from build123d import *

# Parameters (mm, degrees)
F2_R = 1.99999
F3_R = 9


# Not quite as in the source:
# - a fillet or chamfer is up to 0.001 mm smaller than in the source, because OpenCascade refuses the exact size


with BuildPart() as f1:
    # F0 (on Front) → F1 (revolve)
    with BuildSketch(Plane.XZ):
        Polygon((-9.5, -13.2402114049), (-7.5, 23.7597885951), (0, 23.7597885951), (0, 28.8208965212), (-11.5044763215, 28.8208965212), (-11.5044763215, 23.7850059011), (-13.4568578627, -12.3340526108), align=None)
    revolve(axis=Axis((0, 0, 3.3093634993), (0, 0, -1)))

    # F2 (radius 2 in the source; OpenCascade refuses exactly that, so slightly less here)
    f2_edges = [f1.edges().sort_by_distance(p)[0] for p in [
        (9.5, 0, -13.240211),
        (13.456858, 0, -12.334053),
    ]]
    fillet(f2_edges, radius=F2_R)

    # F3
    f3_edges = [f1.edges().sort_by_distance(p)[0] for p in [
        (11.504476, 0, 28.820897),
    ]]
    fillet(f3_edges, radius=F3_R)


solid = f1.part
Check sheet for the modelled part. Datum: model origin and axes. Units: mm. Give positions to 0.01 mm unless a question says otherwise; leave off trailing zeros. Write each loop counter-clockwise with the first axis right and the second up, starting at its lowest first coordinate (ties: lowest second). Pieces come first, ordered by that corner, then holes. Notation, with made-up numbers: (86.25, 74) -> (92.25, 74) arc R18 cw to (92.25, 91) -> close; hole circle Ø9 at (68.5, 74). An arc over 180 degrees is marked (long way). Write item = value, one per line.
Item 1: Sectioned sample at A-A on z = -3.5. Record the boundary of the cut face in (x, y).
Output:
outline = circle Ø25.96 at (0, 0); hole circle Ø17.95 at (0, 0)
Item 2: Gauge pin test, flat ends, axial feed: pin 1 (1 mm diameter, centred on x = -1.5, z = -2, fed in from +Y); pin 2 (2 mm diameter, centred on x = 5, z = -8, fed in from -Y); pin 3 (6 mm diameter, centred on x = -9, z = -7, fed in from -Y). Record the tip position at first contact, or that the pin passes through.
Output:
pin_1 = 12.87
pin_2 = -12.61
pin_3 = -11.73
Item 3: Release check for a two-part mould opening along Y. For faces 1 (the conical face through (-8.034, 2.53, 6.688)), 2 (the conical face through (2.719, -12.243, 4.61)), 3 (the flat face through (0, 0, 28.821)) record: +Y half, -Y half, draft (parallel to the pull), parting line (faces both ways), or undercut.
Output:
face_1 = undercut
face_2 = parting line
face_3 = draft
Item 4: Scan lines: probe 1 along Y at (x, z) = (7.25, -9.5); probe 2 along Y at (x, z) = (0, 5.5); probe 3 along X at (y, z) = (0.5, 10). Record each from-to range of solid material in increasing order. Write a range as from..to.
Output:
probe_1 = -11.15..-5.82, 5.82..11.15
probe_2 = -12.49..-8.49, 8.49..12.49
probe_3 = -12.24..-8.23, 8.23..12.24
Item 5: Sectioned sample at B-B on z = -8.5. Record the boundary of the cut face in (x, y), and give its area (3 significant figures).
Output:
outline = circle Ø26.5 at (0, 0); hole circle Ø18.49 at (0, 0)
area = 283 mm^2
